from build123d import *

# Parameters (mm, degrees)
F0_R     = 6.35
F1_DEPTH = 16.764
F2_R     = 6.35
F2_W     = 27.6436659317
F2_H     = 72.136
F3_DEPTH = 9.652
F4_W     = 13.8218329659
F4_H     = 41.148
F5_DEPTH = 74.676
F7_DEPTH = 53.04913


with BuildPart() as f1:
    # F0 (on Top) → F1 (new body)
    with BuildSketch(Plane.XY):
        Polygon((58.0747899478, -10.0489559141), (-48.8168759839, -10.0489559141), (-48.8168759839, -76.2), (-23.4168759839, -76.2), (58.0747899478, -14.224), align=None)
        with Locations((-26.856459501, -59.436)):
            Circle(F0_R, mode=Mode.SUBTRACT)
        with Locations((-29.5022924669, -21.336)):
            Circle(F0_R, mode=Mode.SUBTRACT)
        with Locations((21.0331240161, -21.336)):
            Circle(F0_R, mode=Mode.SUBTRACT)
    extrude(amount=F1_DEPTH)

    # F2 (on face) → F3 (join)
    with BuildSketch(Plane(origin=(0, -10.0489559141, 0), x_dir=(-1, 0, 0), z_dir=(0, 1, 0))):
        Polygon((-58.0747899478, 16.764), (-58.0747899478, 0), (48.8168759839, 0), (48.8168759839, 16.764), (9.1928759839, 16.764), (-18.4507899478, 16.764), align=None)
        Polygon((-58.0747899478, 101.6), (-58.0747899478, 16.764), (-18.4507899478, 16.764), (-18.4507899478, 88.9), (9.1928759839, 88.9), (9.1928759839, 16.764), (48.8168759839, 16.764), (48.8168759839, 101.6), align=None)
        with Locations((-39.0247899478, 76.2)):
            Circle(F2_R, mode=Mode.SUBTRACT)
        with Locations((29.7668759839, 76.2)):
            Circle(F2_R, mode=Mode.SUBTRACT)
        with Locations((-4.6289569819, 52.832)):
            Rectangle(F2_W, F2_H)
    extrude(amount=F3_DEPTH)

    # F4 (on face) → F5 (join)
    with BuildSketch(Plane.XY.offset(16.764)):
        with Locations((-2.281959501, -30.6229559141)):
            Rectangle(F4_W, F4_H)
    extrude(amount=F5_DEPTH)

    # F6 (on face) → F7 (cut)
    with BuildSketch(Plane.YZ.offset(4.6289569819)):
        Polygon((-51.1969559141, 91.44), (-51.1969559141, 16.764), (-10.0489559141, 91.44), align=None)
    extrude(amount=-F7_DEPTH, mode=Mode.SUBTRACT)


solid = f1.part
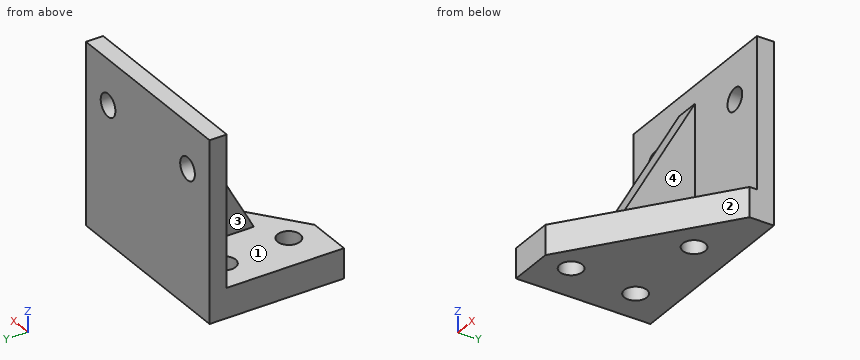
Source: CAD feature listing. Evaluate the final solid. Frame: model axes, mm. Face numbers are marked on the shaded views. A direction names the side the tool comes from. Round coordinates to 2 decimals unless told otherwise and drop trailing zeros. Order: outer loops, then holes, each group sorted by start corner. A loop starts at its lowest first (then second) coordinate and runs counter-clockwise, first axis right, second up. Notation, with made-up numbers: (60.25, 27) - (118.25, 27) arc R21 cw to (118.25, 51) - close; hole circle Ø9 at (88.5, 36.5). An arc over 180 degrees is marked (long way). Use a Markdown table: item, result. Add a question column.
1. Section query D-D (z = 18.5). Return the cut outline in (x, y).
2. Set-up query: the marked faces 1, 2, 3 and 4. Return all of +Z, -Z, +X, -X, +Y, -Y with unobstructed straight access to the full face (end or side cutting, diameter ignored); none if empty.
3. First-contact query: pin 1 (5 mm diameter, centred on x = -24.5, y = -29, fed in from +Z); pin 2 (5 mm diameter, centred on x = -13, y = -46, fed in from -Z); pin 3 (10 mm diameter, centred on x = 39.02, z = 76.2, fed in from +Y) (3 decimals); pin 4 (2 mm diameter, centred on x = -3, z = 63.5, fed in from -Y). Flat tips, straight axial feed; report the tip coordinate or a pass-through.
4. Section query C-C (x = -15). Return the cut outline in (y, z), then the cut area to 3 significant figures.
5. Section query A-A (z = 76.2). Return the cut outline in (x, y), then the cut area to 3 significant figures.
6. Line query: probe 1 along Y at (x, z) = (32, 49); probe 2 along Z at (x, y) = (-44, -23); probe 3 along X at (y, z) = (-21.5, 34). Output: solid intervals per line, ascending.
7. Section query B-B (y = -17.5). Return the cut outline in (x, z).
Derived:
| question | item | result |
|---|---|---|
| 1 | outline | (-48.82, -10.05) - (-9.19, -10.05) - (-9.19, -50.24) - (4.63, -50.24) - (4.63, -10.05) - (58.07, -10.05) - (58.07, -0.4) - (-48.82, -0.4) - close |
| 2 | face 1 | +Z, -Y |
| 2 | face 2 | +Z, -Z, +X, -Y |
| 2 | face 3 | +Z, -X, -Y |
| 2 | face 4 | +Z, +X, -Y |
| 3 | pin 1 | z = 16.76 |
| 3 | pin 2 | z = 0 |
| 3 | pin 3 | through |
| 3 | pin 4 | y = -26 |
| 4 | outline | (-69.8, 0) - (-0.4, 0) - (-0.4, 101.6) - (-10.05, 101.6) - (-10.05, 16.76) - (-69.8, 16.76) - close |
| 4 | area | 1,980 mm2 |
| 5 | outline | (-48.82, -10.05) - (-36.12, -10.05) - (-36.12, -0.4) - (-48.82, -0.4) - close; (-23.42, -10.05) - (-9.19, -10.05) - (-9.19, -18.45) - (4.63, -18.45) - (4.63, -10.05) - (32.67, -10.05) - (32.67, -0.4) - (-23.42, -0.4) - close; (45.37, -10.05) - (58.07, -10.05) - (58.07, -0.4) - (45.37, -0.4) - close |
| 5 | area | 903 mm2 |
| 6 | probe 1 | -10.05 to -0.4 |
| 6 | probe 2 | 0 to 16.76 |
| 6 | probe 3 | -9.19 to 4.63 |
| 7 | outline | (-48.82, 0) - (-34.56, 0) - (-34.56, 16.76) - (-48.82, 16.76) - close; (-24.44, 0) - (15.97, 0) - (15.97, 16.76) - (4.63, 16.76) - (4.63, 77.92) - (-9.19, 77.92) - (-9.19, 16.76) - (-24.44, 16.76) - close; (26.09, 0) - (53.77, 0) - (53.77, 16.76) - (26.09, 16.76) - close |
